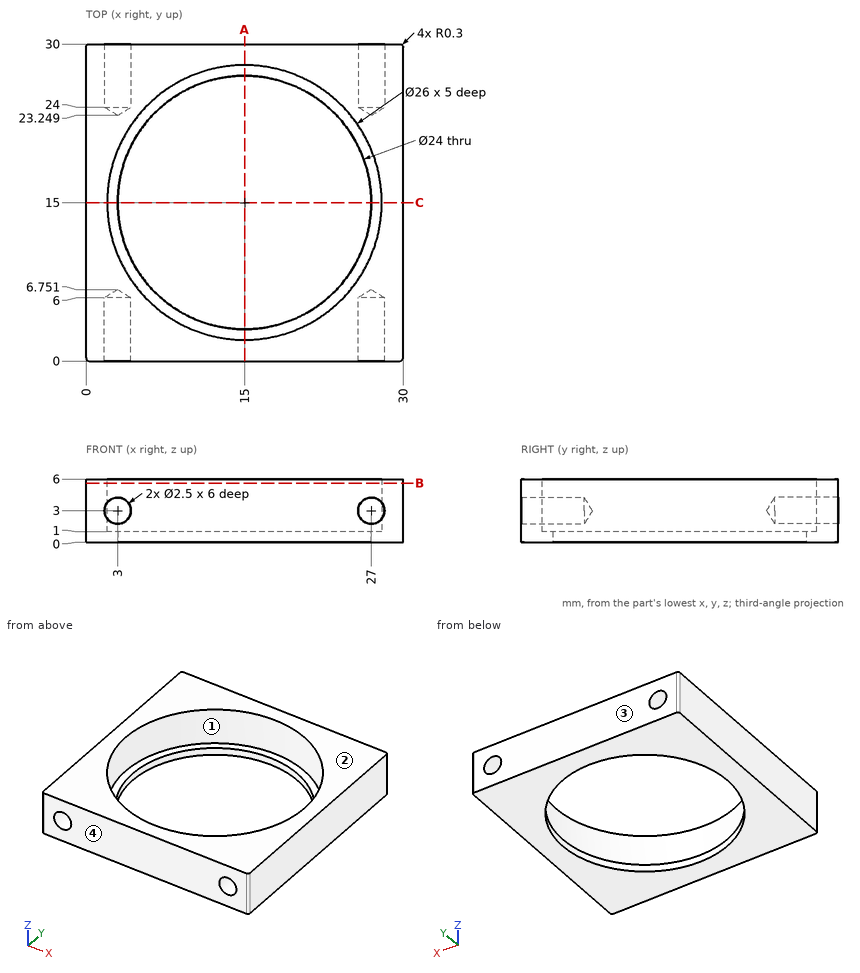
Print and shaded views of the part. All mm, measured from the part's lowest x, y and z. Give positions to 0.01 mm unless a question says otherwise; leave off trailing zeros. Loops run counter-clockwise (first coordinate to the right, second up) from the corner with the lowest first, then second, coordinate; pieces in that order, holes last. Notation, with made-up numbers: (69, 34) -> (112, 34) arc R19 ccw to (112, 64) -> close; hole circle Ø6 at (-8.75, 76.5). An arc over 180 degrees is marked (long way). Use CSV: the item, a comma, the result in double quotes. Start each with the question number.
1) Mould opens along Y. For the marked faces 1, 2, 3 and 4 say: released by +Y, released by -Y, zero draft, split by the parting line, or undercut.
2) Slice it at B-B on z = 5.6. Give the cut face in (x, y).
3) Flat gauge pins, fed straight in: pin 1 Ø2 at (x, z) = (3, 3) entering from +Y; pin 2 Ø2 at (x, z) = (27, 3) entering from -Y. Where does each tip first touch, or does it go through?
4) Wall check: line 1 (Z direction, x = 3, y = 1.6); line 2 (Y direction, x = 15, z = 2.5); line 3 (X direction, y = 15, z = 0.45). Give the ranges that are in metal, low to high.
5) Slice it at A-A on x = 15. Give the cut face in (y, z), plus the area to 3 significant figures.
Computed values:
1,face 1,"undercut"
1,face 2,"zero draft"
1,face 3,"released by +Y"
1,face 4,"released by -Y"
2,outline,"(0, 0.3) arc R0.3 ccw to (0.3, 0) -> (29.7, 0) arc R0.3 ccw to (30, 0.3) -> (30, 29.7) arc R0.3 ccw to (29.7, 30) -> (0.3, 30) arc R0.3 ccw to (0, 29.7) -> close; hole circle Ø26 at (15, 15)"
3,pin 1,"stops at y = 23.85"
3,pin 2,"stops at y = 6.15"
4,line 1,"z = 0 to 1.75, 4.25 to 6"
4,line 2,"y = 0 to 2, 28 to 30"
4,line 3,"x = 0 to 3, 27 to 30"
5,outline,"(0, 0) -> (3, 0) -> (3, 1) -> (2, 1) -> (2, 6) -> (0, 6) -> close; (27, 0) -> (30, 0) -> (30, 6) -> (28, 6) -> (28, 1) -> (27, 1) -> close"
5,area,"26.0 mm^2"
